For this review, take the finished solid that the model builds, in its own axes (mm). A direction names the side the tool comes from. Coordinates: 2 decimals unless noted, no trailing zeros. Loops run counter-clockwise (first coordinate to the right, second up) from the corner with the lowest first, then second, coordinate; pieces in that order, holes last. Notation, with made-up numbers: M 69.5,7.5 L 128.5,7.5 A20 ccw 128.5,26.5 Z; hole C 41.5,-17.75 d4. An arc over 180 degrees is marked long. Write each question's results on one line, items separated by ' | '. Start each with the question number.
```python
from build123d import *

# Parameters (mm, degrees)
SKETCH1_W           = 750
SKETCH1_H           = 750
SKETCH1_W_2         = 710
SKETCH1_H_2         = 710
BOSS_EXTRUDE1_DEPTH = 20
SKETCH2_W           = 20
SKETCH2_H           = 20
BOSS_EXTRUDE2_DEPTH = 710
SKETCH3_W           = 710
SKETCH3_H           = 710
BOSS_EXTRUDE3_DEPTH = 20


with BuildPart() as part:
    # Sketch1 → Boss-Extrude1 (new body)
    with BuildSketch(Plane(origin=(0, 0, 0), x_dir=(1, 0, 0), z_dir=(0, 1, 0))):
        with Locations((375, 375)):
            Rectangle(SKETCH1_W, SKETCH1_H)
        with Locations((375, 375)):
            Rectangle(SKETCH1_W_2, SKETCH1_H_2, mode=Mode.SUBTRACT)
    extrude(amount=BOSS_EXTRUDE1_DEPTH)

    # Sketch2 → Boss-Extrude2 (add)
    with BuildSketch(Plane(origin=(0, 20, 0), x_dir=(1, 0, 0), z_dir=(0, 1, 0))):
        with Locations((10, 740)):
            Rectangle(SKETCH2_W, SKETCH2_H)
        with Locations((740, 740)):
            Rectangle(SKETCH2_W, SKETCH2_H)
        with Locations((10, 10)):
            Rectangle(SKETCH2_W, SKETCH2_H)
        with Locations((740, 10)):
            Rectangle(SKETCH2_W, SKETCH2_H)
    extrude(amount=BOSS_EXTRUDE2_DEPTH)

    # Sketch3 → Boss-Extrude3 (add)
    with BuildSketch(Plane(origin=(0, 730, 0), x_dir=(1, 0, 0), z_dir=(0, 1, 0))):
        Polygon((730, 750), (20, 750), (0, 750), (0, 730), (0, 20), (0, 0), (20, 0), (730, 0), (750, 0), (750, 20), (750, 730), (750, 750), align=None)
        with Locations((375, 375)):
            Rectangle(SKETCH3_W, SKETCH3_H, mode=Mode.SUBTRACT)
    extrude(amount=BOSS_EXTRUDE3_DEPTH)


solid = part.part
```
Q1. Take a section at A-A, the plane x = 180.5. Give the boundary of the cut face in (y, z).
Q2. The part is to be moulded in two halves that separate along X. For faces 6 (the face through (0, 734, -405)), 7 (the face through (20, 10, -370)), 8 (the face through (740, 730, -380)), say which applies: pulls with the +X half, pulls with the -X half, needs draft (parallel to the pull), parting line crosses it, or undercut.
Q3. Insertion check: P1, Ø22, axis at y = 11.5, z = -541.5, coming from the -X side. The pin has a flat end and moves straight along its axis. Give the tip position at first contact, or say it passes through.
Q4. For faces 1 (the face through (405, 734, -750)), 2 (the face through (370, 20, -740)), 3 (the face through (345, 0, -16)), 4 (the face through (370, 10, -730)), 5 (the face through (740, 370, -730)), list the 3-axis set-ups (+Z, -Z, +X, -X, +Y, -Y) from which the entire face can be reached by the end or side of a thin tool; tool diameter is ignored.
Results:
1) outline: M 0,-750 L 20,-750 L 20,-730 L 0,-730 Z; M 0,-20 L 20,-20 L 20,0 L 0,0 Z; M 730,-750 L 750,-750 L 750,-730 L 730,-730 Z; M 730,-20 L 750,-20 L 750,0 L 730,0 Z
2) face 6: pulls with the -X half | face 7: undercut | face 8: needs draft
3) P1: x = 0
4) face 1: -Z, +X, -X, +Y, -Y | face 2: +Z, -Z | face 3: +Z, -Z, +X, -X, -Y | face 4: +Y, -Y | face 5: +X, -X
